Read the model definition and answer for the solid it produces. Units are mm, in the model's axes. A direction names the side the tool comes from. Coordinates: 2 decimals unless noted, no trailing zeros. Order: outer loops, then holes, each group sorted by start corner. A loop starts at its lowest first (then second) coordinate and runs counter-clockwise, first axis right, second up. Notation, with made-up numbers: M -13.75,-12.5 L 22.25,-12.5 A8 ccw 22.25,-5.5 Z; hole C -35,16 d3. An arc over 180 degrees is marked long. Write each question's results on one line, items separated by ' | '.
```python
from build123d import *

# Parameters (mm, degrees)
F1_DEPTH = 25
F2_R     = 5
F3_DEPTH = 5


with BuildPart() as f1:
    # F0 (on Front) → F1 (new body)
    with BuildSketch(Plane.XZ):
        with BuildLine():
            ThreePointArc((25.259304, -18.427804), (29.960421, -9.741836), (31.586196, 0))
            ThreePointArc((31.586196, 0), (-7.638587, 28.546513), (-22.740696, -17.555692))
            Line((-22.740696, -17.555692), (25.259304, -17.555692))
            Line((25.259304, -17.555692), (25.259304, -18.427804))
        make_face()
        with BuildLine():
            Line((25.259304, -17.555692), (-22.740696, -17.555692))
            ThreePointArc((-22.740696, -17.555692), (1.041216, -29.99505), (25.259304, -18.427804))
            Line((25.259304, -18.427804), (25.259304, -17.555692))
        make_face()
        with BuildLine():
            ThreePointArc((25.259304, -18.427804), (1.041216, -29.99505), (-22.740696, -17.555692))
            Line((-22.740696, -17.555692), (-22.740696, -317.555692))
            Line((-22.740696, -317.555692), (25.259304, -317.555692))
            Line((25.259304, -317.555692), (25.259304, -18.427804))
        make_face()
    extrude(amount=F1_DEPTH)

    # F2 (on face) → F3 (cut)
    with BuildSketch(Plane(origin=(0, 0, 0), x_dir=(-1, 0, 0), z_dir=(0, 1, 0))):
        Circle(F2_R)
    extrude(amount=-F3_DEPTH, mode=Mode.SUBTRACT)


solid = f1.part
```
(1) For faces 4 (the flat face through (-22.741, -12, -165)), 5 (the cylindrical face through (1.08, -2.46, -4.88)), 6 (the flat face through (1, -25, -141)), determine the directions among +Z, -Z, +X, -X, +Y, -Y from which every point of the face is accessible in a straight line to the end or side of a thin tool.
Conclusion:
face 4: -Z, -X, +Y, -Y | face 5: +Y | face 6: +Z, -Z, +X, -X, -Y
(2) The mould has two halves that part along X. Classify faces 1 (the flat face through (0, -5, 0)), 2 (the flat face through (1, -12, -317.556)), 3 (the flat face through (25.259, -12, -170)): pulls with the +X half, pulls with the -X half, needs draft (parallel to the pull), parting line crosses it, or undercut.
Conclusion:
face 1: undercut | face 2: needs draft | face 3: pulls with the +X half
(3) Straight lines are drawn through the part: line 1 (Z direction, x = 0, y = -2.45); line 2 (X direction, y = -22, z = -115.5); line 3 (Z direction, x = 1.5, y = -5.5). For each, find the intervals that lie inside material, in ascending order.
Conclusion:
line 1: -317.56 to -5, 5 to 29.96 | line 2: -22.74 to 25.26 | line 3: -317.56 to 30
(4) The part is cut by section C-C, the plane x = 20.5. Write down the section's boundary in (y, z), then the cut area to 3 significant figures.
Conclusion:
outline: M -25,-317.56 L 0,-317.56 L 0,23.29 L -25,23.29 Z | area: 8,520 mm²
(5) The part is cut by section A-A, the plane y = -19. Write down the section's boundary in (x, z), then the cut area to 3 significant figures.
Conclusion:
outline: M -22.74,-317.56 L 25.26,-317.56 L 25.26,-18.43 A30 ccw 31.59,0 A30 ccw long -22.74,-17.56 Z | area: 16,800 mm²
(6) The part is cut by section B-B, the plane z = -57. Write down the section's boundary in (x, y).
Conclusion:
outline: M -22.74,-25 L 25.26,-25 L 25.26,0 L -22.74,0 Z
(7) Given pin 1 (12.5 mm diameter, centred on y = -13, z = -127.5, fed in from +X); pin 2 (6 mm diameter, centred on y = -7, z = -250, fed in from -X); pin 3 (10 mm diameter, centred on x = -21.5, y = -9.5, fed in from +Z), each flat-ended and moving along its own axis, determine where each tip first touches the part or whether it passes through.
Conclusion:
pin 1: x = 25.26 | pin 2: x = -22.74 | pin 3: z = 23.94
